Source: CAD feature listing. Evaluate the final solid. Frame: model axes, mm. Face numbers are marked on the shaded views. A direction names the side the tool comes from. Coordinates: 2 decimals unless noted, no trailing zeros. Write each loop counter-clockwise with the first axis right and the second up, starting at its lowest first coordinate (ties: lowest second). Pieces come first, ordered by that corner, then holes. Notation, with made-up numbers: (24.5, -37.5) -> (43.5, -37.5) arc R14 cw to (43.5, -13.5) -> close; hole circle Ø6 at (37, 11). An arc over 180 degrees is marked (long way). One line per item, written item: value. Start each with the question number.
1. Line query: line 1 (X direction, y = -4, z = -25); line 2 (X direction, y = 7, z = -22); line 3 (X direction, y = 0, z = -26). Output: solid intervals per line, ascending.
2. Section query B-B, the plane x = 40.5. Output: boundary loops of the cut face in (y, z).
3. Access query for the marked faces 1, 2, 3 and 4. Directions: +Z, -Z, +X, -X, +Y, -Y. A direction counts if a zero-diameter tool reaches every point of the face in a straight line with its end or side. Return the directions, or none.
4. First-contact query: P1, Ø10, axis at y = 0, z = 0, coming from the -X side; P2, Ø8, axis at x = 13, y = 16.5, coming from the -Z side; P3, Ø7, axis at x = 68.072, z = -25.4, coming from the -Y side; P4, Ø8.5, axis at x = -37.5, z = -1.5, coming from the -Y side. Flat tips, straight axial feed; report the tip coordinate or a pass-through.
5. Section query A-A, the plane y = -17.78. Output: boundary loops of the cut face in (x, z) (3 decimals).
6. Section query D-D, the plane z = 25.4. Output: boundary loops of the cut face in (x, y).
7. Section query C-C, the plane z = -25.4. Output: boundary loops of the cut face in (x, y).
from build123d import *

# Parameters (mm, degrees)
SKETCH1_W          = 63.5
SKETCH1_H          = 50.8
EXTRUDE1_DEPTH     = 95.25
SKETCH5_R          = 22.225
EXTRUDE2_DEPTH     = 5.969
SKETCH6_W          = 14.2875
SKETCH6_H          = 35.56
CUT_EXTRUDE4_DEPTH = 30.48
HOLE1_D            = 8.7376
HOLE1_DEPTH        = 95.25
HOLE2_D            = 8.7376
HOLE2_DEPTH        = 50.8
LPATTERN1_COUNT    = 2
LPATTERN1_PITCH    = 41.275


with BuildPart() as part:
    # Sketch1 → Extrude1 (new body)
    with BuildSketch(Plane(origin=(0, 0, 0), x_dir=(0, 0, -1), z_dir=(1, 0, 0))):
        Rectangle(SKETCH1_W, SKETCH1_H)
    extrude(amount=EXTRUDE1_DEPTH)

    # S2D0002 → Cut-Revolve1 (revolve, cut)
    with BuildSketch(Plane(origin=(0, 17.4752, 0), x_dir=(-1, 0, 0), z_dir=(0, 1, 0)), mode=Mode.PRIVATE) as cut_revolve1_sk:
        Polygon((-18.8849, -31.496), (-22.225, -31.496), (-22.225, -31.75), (-12.7, -31.75), (-12.7, -17.526), (-17.6784, -17.526), (-17.6784, -28.279393135), (-18.342306865, -28.9433), align=None)
    revolve(cut_revolve1_sk.sketch.rotate(Axis((12.7, 17.4752, -19.13842003), (0, 0, 1)), 180), axis=Axis((12.7, 17.4752, -19.13842003), (0, 0, 1)), mode=Mode.SUBTRACT)  # turned: the seam where the file's is

    # Sketch3 → Cut-Revolve2 (revolve, cut)
    with BuildSketch(Plane(origin=(41.148, 0, -25.146), x_dir=(1, 0, 0), z_dir=(0, 1, 0))):
        Polygon((45.1993, 6.35), (48.5394, 6.35), (48.5394, 6.604), (39.0144, 6.604), (39.0144, -7.62), (43.9928, -7.62), (43.9928, 3.133393135), (44.656706865, 3.7973), align=None)
    revolve(axis=Axis((80.1624, 0, -3.189624441), (0, 0, -1)), mode=Mode.SUBTRACT)

    # Sketch4 → Cut-Revolve3 (revolve, cut)
    with BuildSketch(Plane(origin=(53.975, 0, 0), x_dir=(0, -1, 0), z_dir=(0, 0, 1)), mode=Mode.PRIVATE) as cut_revolve3_sk:
        Polygon((6.1849, 38.227), (9.525, 38.227), (9.525, 41.275), (0, 41.275), (0, 26.8732), (4.9784, 26.8732), (4.9784, 35.010393135), (5.642306865, 35.6743), align=None)
    revolve(cut_revolve3_sk.sketch.rotate(Axis((38.879609832, 0, 0), (1, 0, 0)), 270), axis=Axis((38.879609832, 0, 0), (1, 0, 0)), mode=Mode.SUBTRACT)  # turned: the seam where the file's is

    # Sketch5 → Extrude2 (add)
    with BuildSketch(Plane.ZY):
        Circle(SKETCH5_R)
    extrude(amount=EXTRUDE2_DEPTH)

    # Sketch6 → Revolve1 (revolve)
    with BuildSketch(Plane(origin=(0, 0, 0), x_dir=(0, 0, 1), z_dir=(0, -1, 0)), mode=Mode.PRIVATE) as revolve1_sk:
        with Locations((-7.14375, 23.749)):
            Rectangle(SKETCH6_W, SKETCH6_H)
    revolve(revolve1_sk.sketch.rotate(Axis((5.754582971, 0, 0), (-1, 0, 0)), 180), axis=Axis((5.754582971, 0, 0), (-1, 0, 0)))  # turned: the seam where the file's is

    # S2D0001 → Cut-Revolve4 (revolve, cut)
    with BuildSketch(Plane(origin=(-18.511260017, 3.2639, 0), x_dir=(0, 1, 0), z_dir=(0, 0, 1)), mode=Mode.PRIVATE) as cut_revolve4_sk:
        Polygon((2.286, 20.950017728), (2.286, 6.634739983), (-3.2639, 6.634739983), (-3.2639, 23.017739983), (3.4798, 23.017739983), align=None)
    revolve(cut_revolve4_sk.sketch.rotate(Axis((0, 0, 0), (-1, 0, 0)), 270), axis=Axis((0, 0, 0), (-1, 0, 0)), mode=Mode.SUBTRACT)  # turned: the seam where the file's is

    # Sketch8 → Cut-Revolve5 (revolve, cut)
    with BuildSketch(Plane(origin=(0, 0, 0), x_dir=(0, 0, -1), z_dir=(0, 1, 0)), mode=Mode.PRIVATE) as cut_revolve5_sk:
        with BuildLine():
            Line((-14.2875, 31.623), (-14.097, 32.385))
            Line((-14.097, 32.385), (-14.097, 40.513))
            ThreePointArc((-14.097, 40.513), (-13.996678675, 41.056796865), (-13.708922533, 41.529))
            Line((-13.708922533, 41.529), (-14.2875, 41.529))
            Line((-14.2875, 41.529), (-14.2875, 31.623))
        make_face()
    revolve(cut_revolve5_sk.sketch.rotate(Axis((-12.65936, 0, 0), (-1, 0, 0)), 180), axis=Axis((-12.65936, 0, 0), (-1, 0, 0)), mode=Mode.SUBTRACT)  # turned: the seam where the file's is

    # Sketch12 → Cut-Extrude4 (cut, symmetric)
    with BuildSketch(Plane(origin=(0, 0, 0), x_dir=(0, -1, 0), z_dir=(0, 0, -1))):
        Polygon((12.573, 41.529), (12.573, 33.9598), (14.097, 32.4358), (14.097, 41.529), align=None)
        Polygon((-12.573, 41.529), (-12.573, 33.9598), (-14.097, 32.4358), (-14.097, 41.529), align=None)
    extrude(amount=CUT_EXTRUDE4_DEPTH, both=True, mode=Mode.SUBTRACT)

    # Hole1
    with Locations(Plane.ZY):
        with Locations((-24.13, -17.78), (24.13, 17.78)):
            Hole(HOLE1_D / 2, depth=HOLE1_DEPTH)

    # Hole2
    with Locations(Plane(origin=(0, 25.4, 0), x_dir=(-1, 0, 0), z_dir=(0, 1, 0))):
        with Locations((-26.797, -25.4), (-26.797, 25.4)):
            hole2 = Hole(HOLE2_D / 2, depth=HOLE2_DEPTH)

    # LPattern1: Hole2 ×2
    with Locations(*[(i * LPATTERN1_PITCH, 0, 0) for i in range(1, LPATTERN1_COUNT)]):
        add(hole2, mode=Mode.SUBTRACT)


solid = part.part
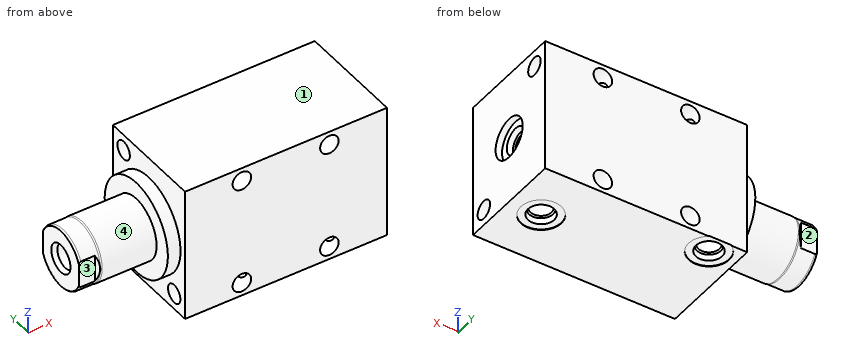
Computed values:
1. line 1: x = 0 to 22.45, 31.15 to 63.72, 72.42 to 77.2, 83.13 to 95.25
1. line 2: x = 0 to 24.05, 29.54 to 65.33, 70.82 to 95.25
1. line 3: x = 0 to 22.47, 31.12 to 63.74, 72.4 to 75.18, 85.14 to 95.25
2. outline: (-25.4, -31.75) -> (25.4, -31.75) -> (25.4, 31.75) -> (-25.4, 31.75) -> close; hole circle Ø8.74 at (-17.78, -24.13); hole circle Ø8.74 at (17.78, 24.13)
3. face 1: +Z, +X, -X, +Y, -Y
3. face 2: +Z, -Z, -X, +Y
3. face 3: +Z, -Z, -X, -Y
3. face 4: -X
4. P1: stops at x = -25.15
4. P2: stops at z = -28.32
4. P3: passes through
4. P4: stops at y = -13.28
5. outline: (-5.969, -13.335) -> (0, -13.335) -> (0, -19.761) -> (95.25, -19.761) -> (95.25, 31.75) -> (0, 31.75) -> (0, 13.335) -> (-5.969, 13.335) -> close; (0, -31.75) -> (95.25, -31.75) -> (95.25, -28.499) -> (71.152, -28.499) arc R4.369 cw to (64.992, -28.499) -> (29.877, -28.499) arc R4.369 cw to (23.717, -28.499) -> (0, -28.499) -> close; hole circle Ø8.738 at (26.797, 25.4); hole circle Ø8.738 at (68.072, 25.4)
6. outline: (0, -25.4) -> (22.43, -25.4) -> (22.43, 13.6) -> (0, 13.6) -> close; (0, 21.96) -> (22.43, 21.96) -> (22.43, 25.4) -> (0, 25.4) -> close; (31.17, -25.4) -> (63.7, -25.4) -> (63.7, 13.6) -> (31.17, 13.6) -> close; (31.17, 21.96) -> (63.7, 21.96) -> (63.7, 25.4) -> (31.17, 25.4) -> close; (72.44, -25.4) -> (95.25, -25.4) -> (95.25, 13.6) -> (72.44, 13.6) -> close; (72.44, 21.96) -> (95.25, 21.96) -> (95.25, 25.4) -> (72.44, 25.4) -> close
7. outline: (0, -25.4) -> (22.43, -25.4) -> (22.43, -21.96) -> (0, -21.96) -> close; (0, -13.6) -> (22.43, -13.6) -> (22.43, 25.4) -> (0, 25.4) -> close; (31.17, -25.4) -> (63.7, -25.4) -> (63.7, -21.96) -> (31.17, -21.96) -> close; (31.17, -13.6) -> (63.7, -13.6) -> (63.7, 25.4) -> (31.17, 25.4) -> close; (72.44, -25.4) -> (95.25, -25.4) -> (95.25, -21.96) -> (72.44, -21.96) -> close; (72.44, -13.6) -> (95.25, -13.6) -> (95.25, 25.4) -> (72.44, 25.4) -> close; hole circle Ø9.96 at (12.7, 17.48); hole circle Ø9.96 at (80.16, 0)
